from build123d import *

# Parameters (mm, degrees)
SKETCH1_W           = 133.500000388
SKETCH1_H           = 84
BOSS_EXTRUDE1_DEPTH = 3
SKETCH2_W           = 20
SKETCH2_H           = 3
CUT_EXTRUDE1_DEPTH  = 104.014399147
SKETCH3_W           = 3
SKETCH3_H           = 30
BOSS_EXTRUDE2_DEPTH = 3
SKETCH4_W           = 3
SKETCH4_H           = 3.4
CUT_EXTRUDE2_DEPTH  = 106.612611798
SKETCH6_W           = 20
SKETCH6_H           = 35.000000221
CUT_EXTRUDE3_DEPTH  = 106.612611798


with BuildPart() as part:
    # Sketch1 → Boss-Extrude1 (new body)
    with BuildSketch(Plane(origin=(0, 0, 0), x_dir=(1, 0, 0), z_dir=(0, 1, 0))):
        with Locations((22.092889694, -10.056770433)):
            Rectangle(SKETCH1_W, SKETCH1_H)
    extrude(amount=BOSS_EXTRUDE1_DEPTH)

    # Sketch2 → Cut-Extrude1 (cut, through all)
    with BuildSketch(Plane.XZ):
        with Locations((63.842889888, 46.556770433)):
            Rectangle(SKETCH2_W, SKETCH2_H)
        with Locations((-19.6571105, 46.556770433)):
            Rectangle(SKETCH2_W, SKETCH2_H)
        with Locations((-19.6571105, -26.443229567)):
            Rectangle(SKETCH2_W, SKETCH2_H)
        with Locations((63.842889888, -26.443229567)):
            Rectangle(SKETCH2_W, SKETCH2_H)
    extrude(amount=-CUT_EXTRUDE1_DEPTH, mode=Mode.SUBTRACT)

    # Sketch3 → Boss-Extrude2 (add, through all)
    with BuildSketch(Plane.XZ):
        with Locations((90.342889888, 10.056770433)):
            Rectangle(SKETCH3_W, SKETCH3_H)
        with Locations((-46.1571105, 10.056770433)):
            Rectangle(SKETCH3_W, SKETCH3_H)
    extrude(amount=-BOSS_EXTRUDE2_DEPTH)

    # Sketch4 → Cut-Extrude2 (cut, symmetric)
    with BuildSketch(Plane.XZ):
        Polygon((88.842889888, 8.356770433), (88.842889888, 5.056770433), (91.842889888, 5.056770433), (91.842889888, 15.056770433), (88.842889888, 15.056770433), (88.842889888, 11.756770433), align=None)
        with Locations((87.342889888, 10.056770433)):
            Rectangle(SKETCH4_W, SKETCH4_H)
        Polygon((85.842889888, 7.156770433), (85.842889888, 8.356770433), (85.842889888, 11.756770433), (85.842889888, 12.956770433), (82.842889888, 12.956770433), (82.842889888, 11.756770433), (82.842889888, 8.356770433), (82.842889888, 7.156770433), align=None)
        with Locations((81.342889888, 10.056770433)):
            Rectangle(SKETCH4_W, SKETCH4_H)
    cut_extrude2 = extrude(amount=CUT_EXTRUDE2_DEPTH, both=True, mode=Mode.SUBTRACT)

    # Mirror1: Cut-Extrude2 across plane
    add(cut_extrude2.mirror(Plane(origin=(22.092889694, 0, 0), x_dir=(0, 0, 1), z_dir=(1, 0, 0))), mode=Mode.SUBTRACT)

    # Sketch6 → Cut-Extrude3 (cut, through all)
    with BuildSketch(Plane.XZ):
        with Locations((35.292890439, 21.956770364)):
            Rectangle(SKETCH6_W, SKETCH6_H)
    extrude(amount=-CUT_EXTRUDE3_DEPTH, mode=Mode.SUBTRACT)


solid = part.part
Check sheet for the modelled part. Datum: model origin and axes. Units: mm. A direction names the side the tool comes from. Coordinates: 2 decimals unless noted, no trailing zeros. Write each loop counter-clockwise with the first axis right and the second up, starting at its lowest first coordinate (ties: lowest second). Pieces come first, ordered by that corner, then holes. Notation, with made-up numbers: M -16,-2.75 L 29,-2.75 A19 cw 29,31.25 Z; hole C 46.5,-2.75 d2. An arc over 180 degrees is marked long. Answer as CSV lines item,"result".
Q1. Mould release check, pull along Z, two halves, no side actions. Record for faces 1 (the face through (-47.657, 1, 0)), 2 (the face through (64, 1, 45.057)), 3 (the face through (64, 1, -24.943)): released by +Z, released by -Z, zero draft, split by the parting line, or undercut.
Check result:
face 1,"zero draft"
face 2,"undercut"
face 3,"undercut"
Q2. Cross-section at A-A (x = 60.5). Record the boundary of the cut face in (y, z), then the cut area to 3 significant figures.
Check result:
outline,"M 0,-31.94 L 3,-31.94 L 3,-27.94 L 0,-27.94 Z; M 0,-24.94 L 3,-24.94 L 3,45.06 L 0,45.06 Z; M 0,48.06 L 3,48.06 L 3,52.06 L 0,52.06 Z"
area,"234 mm^2"
Q3. Set-up check for faces 4 (the face through (-44.657, 1, -18)), 5 (the face through (-37, 1, 11.757)), 6 (the face through (73.843, 1, 47)): record each of +Z, -Z, +X, -X, +Y, -Y from which the full face is reachable in a straight line by a thin tool's end or side.
Check result:
face 4,"-Z, -X, +Y, -Y"
face 5,"-X, +Y, -Y"
face 6,"+Y, -Y"
Q4. Cross-section at D-D (z = 35.5). Record the boundary of the cut face in (x, y), then the cut area to 4 significant figures.
Check result:
outline,"M -44.66,0 L 25.29,0 L 25.29,3 L -44.66,3 Z; M 45.29,0 L 88.84,0 L 88.84,3 L 45.29,3 Z"
area,"340.5 mm^2"
Q5. Go/stop test with flat-tipped pins: pin 1 (1.5 mm diameter, centred on y = 2, z = 14.5, fed in from +X); pin 2 (0.9 mm diameter, centred on y = 1, z = 13, fed in from -X); pin 3 (1.5 mm diameter, centred on y = 1.5, z = 10, fed in from +X). Record where each tip stops, or that it passes through.
Check result:
pin 1,"x = 91.84"
pin 2,"x = -44.66"
pin 3,"x = 79.84"
Q6. Material ranges on probe 1 along X at (y, z) = (2.45, 46.5); probe 2 along Z at (x, y) = (-19, 2.75); probe 3 along Z at (x, y) = (-38, 1.3), recorded low to high. Write a range as from..to.
Check result:
probe 1,"-44.66..-29.66, -9.66..53.84, 73.84..88.84"
probe 2,"-31.94..-27.94, -24.94..45.06, 48.06..52.06"
probe 3,"-31.94..8.36, 11.76..52.06"
Q7. Cross-section at C-C (y = 1.9). Count the separate pieces of the cut face and the enclosed holes in it, then the cut area to 3 significant figures.
Check result:
separate pieces,"1"
enclosed holes,"5"
area,"10,300 mm^2"
Q8. Cross-section at B-B (z = 10). Record the boundary of the cut face in (x, y).
Check result:
outline,"M -35.66,0 L 25.29,0 L 25.29,3 L -35.66,3 Z; M 45.29,0 L 79.84,0 L 79.84,3 L 45.29,3 Z"
